from build123d import *

# Parameters (mm, degrees)
SKETCH014_W          = 14
SKETCH014_H          = 3
PAD006_DEPTH         = 42
SKETCH015_R          = 1.5
POCKET007_DEPTH      = 5
POCKET008_DEPTH      = 2
POCKET008_DEPTH_BACK = 3
SKETCH018_W          = 5
SKETCH018_H          = 15
POCKET009_DEPTH      = 43
SKETCH020_W          = 9.5
SKETCH020_H          = 6.5
PAD008_DEPTH         = 3.85
PAD008_DEPTH_BACK    = 1
SKETCH019_R          = 1.5
POCKET010_DEPTH      = 8
POCKET010_DEPTH_BACK = 100
SKETCH021_W          = 2.25
SKETCH021_H          = 5.5
POCKET011_DEPTH      = 42


with BuildPart() as part:
    # Sketch013 → Revolution (revolve)
    with BuildSketch(Plane.YZ):
        Polygon((10, 0), (14, 0), (14, -42), (12, -42), align=None)
    revolve(axis=Axis((0, 0, 0), (0, 0, 1)))

    # Sketch014 (on Face1 of Revolution) → Pad006 (new body)
    with BuildSketch(Plane(origin=(0, 0, 0), x_dir=(0, -1, 0), z_dir=(0, 0, 1))):
        with Locations((0, 13.5)):
            Rectangle(SKETCH014_W, SKETCH014_H)
    extrude(amount=-PAD006_DEPTH)

    # Sketch015 (on Face11 of Pad006) → Pocket007 (cut)
    with BuildSketch(Plane.YZ.offset(15)):
        with Locations((0, -6)):
            Circle(SKETCH015_R)
        with Locations((0, -18)):
            Circle(SKETCH015_R)
        with Locations((0, -30)):
            Circle(SKETCH015_R)
    extrude(amount=-POCKET007_DEPTH, mode=Mode.SUBTRACT)

    # Sketch016 (on DatumPlane) → Pocket008 (cut, two sides)
    with BuildSketch(Plane(origin=(11.920048, -2.3e-05, -21.627207), x_dir=(-2e-06, -1, 0), z_dir=(-0.999996, 2e-06, -0.003))) as pocket008_sk:
        Polygon((2.75, 14.039346), (2.75, 17.214772), (0, 18.802485), (-2.75, 17.214772), (-2.75, 14.039346), (0, 12.451632), align=None)
        Polygon((2.75, 2.039346), (2.75, 5.214772), (0, 6.802485), (-2.75, 5.214772), (-2.75, 2.039346), (0, 0.451632), align=None)
        Polygon((2.75, -9.960654), (2.75, -6.785228), (0, -5.197515), (-2.75, -6.785228), (-2.75, -9.960654), (0, -11.548368), align=None)
    extrude(amount=-POCKET008_DEPTH, mode=Mode.SUBTRACT)
    extrude(pocket008_sk.sketch, amount=POCKET008_DEPTH_BACK, mode=Mode.SUBTRACT)

    # Sketch018 (on Face1 of Pocket008) → Pocket009 (cut)
    with BuildSketch(Plane(origin=(0, 0, 0), x_dir=(0, -1, 0), z_dir=(0, 0, 1))):
        with Locations((0, -7.5)):
            Rectangle(SKETCH018_W, SKETCH018_H)
    extrude(amount=-POCKET009_DEPTH, mode=Mode.SUBTRACT)

    # Sketch020 (on DatumPlane) → Pad008 (join, two sides)
    with BuildSketch(Plane(origin=(15, 14, 0), x_dir=(-1, 0, 0), z_dir=(0, 1, 0))) as pad008_sk:
        with Locations((15, -6)):
            Rectangle(SKETCH020_W, SKETCH020_H)
        with Locations((15, -36)):
            Rectangle(SKETCH020_W, SKETCH020_H)
    pad008 = extrude(amount=PAD008_DEPTH) + extrude(pad008_sk.sketch, amount=-PAD008_DEPTH_BACK)

    # Mirrored: Pad008 across XZ
    add(pad008.mirror(Plane.XZ))

    # Sketch019 (on DatumPlane) → Pocket010 (cut, two sides)
    with BuildSketch(Plane(origin=(15, 12, 0), x_dir=(1, 0, 0), z_dir=(0, -1, 0))) as pocket010_sk:
        with Locations((-15, -6)):
            Circle(SKETCH019_R)
        with Locations((-15, -36)):
            Circle(SKETCH019_R)
    extrude(amount=-POCKET010_DEPTH, mode=Mode.SUBTRACT)
    extrude(pocket010_sk.sketch, amount=POCKET010_DEPTH_BACK, mode=Mode.SUBTRACT)

    # Sketch021 (on Face17 of Pocket010) → Pocket011 (cut)
    with BuildSketch(Plane.YX.offset(39.25)):
        with Locations((-15.125, 0)):
            Rectangle(SKETCH021_W, SKETCH021_H)
    pocket011 = extrude(amount=-POCKET011_DEPTH, mode=Mode.SUBTRACT)

    # Mirrored001: Pocket011 across XZ
    add(pocket011.mirror(Plane.XZ), mode=Mode.SUBTRACT)


solid = part.part
Check sheet for the modelled part. Datum: model origin and axes. Units: mm. A direction names the side the tool comes from. Round coordinates to 2 decimals unless told otherwise and drop trailing zeros. Order: outer loops, then holes, each group sorted by start corner. A loop starts at its lowest first (then second) coordinate and runs counter-clockwise, first axis right, second up.
Q1. Cross-section at A-A, the plane z = -17. Enter the section's corners in (x, y), plus the area to 3 significant figures.
Filled sheet:
outline: (-13.77, -2.5) arc R14 ccw to (12.12, -7) - (15, -7) - (15, -1.12) - (13.91, -1.12) - (13.91, -2.75) - (10.45, -2.75) arc R10.81 cw to (-10.52, -2.5) - close; (-13.77, 2.5) - (-10.52, 2.5) arc R10.81 cw to (10.45, 2.75) - (13.91, 2.75) - (13.91, 1.12) - (15, 1.12) - (15, 7) - (12.12, 7) arc R14 ccw to start
area: 235 mm2
Q2. Cross-section at B-B, the plane z = -12.5. Enter the section's corners in (x, y).
Filled sheet:
outline: (-13.77, -2.5) arc R14 ccw to (12.12, -7) - (15, -7) - (15, 7) - (12.12, 7) arc R14 ccw to (-13.77, 2.5) - (-10.3, 2.5) arc R10.6 cw (long way) to (-10.3, -2.5) - close
Q3. Draft check along X on faces 1 (the face through (14, -7, -21)), 2 (the face through (-0.195, -12.785, -34.513)). Enter one of: pulls with the +X half, pulls with the -X half, needs draft (parallel to the pull), parting line crosses it, or undercut.
Filled sheet:
face 1: needs draft
face 2: undercut
Q4. Scan lines: L1, parallel to Y at x = 14.45, z = -30; L2, parallel to X at y = 14.5, z = -37; L3, parallel to Y at x = 13, z = -6.5. Record each from-to range of solid material in increasing order.
Filled sheet:
L1: y = -7 to -1.5, 1.5 to 7
L2: x = -4.75 to -2.75, 2.75 to 4.75
L3: y = -7 to -2.75, 2.75 to 7
Q5. Depth check by flat-ended pin: P1, Ø2.5, axis at y = -15.5, z = -36, coming from the +X side; P2, Ø4, axis at y = 9, z = -35.5, coming from the -X side; P3, Ø1.5, axis at y = 10.5, z = -14.5, coming from the +X side; P4, Ø2.5, axis at x = 0, z = -6, coming from the -Y side. Enter the tip coordinate at first touch or a pass-through.
Filled sheet:
P1: stops at x = 4.75
P2: stops at x = -12.12
P3: stops at x = 10.05
P4: passes through
Q6. Cross-section at C-C, the plane z = -30. Enter the section's corners in (x, y).
Filled sheet:
outline: (-13.77, -2.5) arc R14 ccw to (12.12, -7) - (15, -7) - (15, -1.5) - (13.95, -1.5) - (13.95, -2.75) - (11.09, -2.75) arc R11.43 cw to (-11.15, -2.5) - close; (-13.77, 2.5) - (-11.15, 2.5) arc R11.43 cw to (11.09, 2.75) - (13.95, 2.75) - (13.95, 1.5) - (15, 1.5) - (15, 7) - (12.12, 7) arc R14 ccw to start
Q7. Set-up check for faces 3 (the face through (-0.325, 17.039, -7.464)), 4 (the face through (-12, 2.5, -21)), 5 (the face through (-2.75, 15, -36)): record each of +Z, -Z, +X, -X, +Y, -Y from which the full face is reachable in a straight line by a thin tool's end or side.
Filled sheet:
face 3: +Y, -Y
face 4: +Z, -Z, -X
face 5: +Z, -Z
Q8. Cross-section at D-D, the plane z = -6. Give the number of separate pieces and of enclosed holes in the cut face, plus the area to 3 significant figures.
Filled sheet:
separate pieces: 4
enclosed holes: 0
area: 285 mm2
